from build123d import *

# Parameters (mm, degrees)
F0_W = 64.1248
F0_H = 25.463037
F2_T = -1.27
F4_D = 7.62


with BuildPart() as f1:
    # F0 (on Front) → F1 (revolve)
    with BuildSketch(Plane.XZ):
        with Locations((32.0624, 12.731518)):
            Rectangle(F0_W, F0_H)
    revolve(axis=Axis((0, 0, 5.022522), (0, 0, -1)))

    # F2
    f2_openings = [f1.faces().sort_by_distance(p)[0] for p in [
        (0, 0, 25.463037),
    ]]
    offset(amount=F2_T, openings=f2_openings)

    # F4 (through all)
    with Locations(Plane(origin=(0, 0, 0), x_dir=(1, 0, 0), z_dir=(0, 0, -1))):
        with Locations((0, 0)):
            Hole(F4_D / 2)


solid = f1.part
Geometry: final body of the model. Coordinates: model frame, mm. A direction names the side the tool comes from. Give positions to 0.01 mm unless a question says otherwise; leave off trailing zeros. Order: outer loops, then holes, each group sorted by start corner. A loop starts at its lowest first (then second) coordinate and runs counter-clockwise, first axis right, second up. Notation, with made-up numbers: (-29.5, 10.5) -> (-24.5, 10.5) arc R30 ccw to (-24.5, 47.5) -> close; hole circle Ø1 at (33.5, 68). An arc over 180 degrees is marked (long way). Answer as a JSON object with one key per item and string values.
Q1. Section D-D (y = -17.5). Output: boundary loops of the cut face in (x, z), plus the area to 3 significant figures.
Entries:
{"outline": "(-61.69, 0) -> (61.69, 0) -> (61.69, 25.46) -> (60.37, 25.46) -> (60.37, 1.27) -> (-60.37, 1.27) -> (-60.37, 25.46) -> (-61.69, 25.46) -> close", "area": "221 mm^2"}
Q2. Section A-A (x = 0). Output: boundary loops of the cut face in (y, z), plus the area to 3 significant figures.
Entries:
{"outline": "(-64.12, 0) -> (-3.81, 0) -> (-3.81, 1.27) -> (-62.85, 1.27) -> (-62.85, 25.46) -> (-64.12, 25.46) -> close; (3.81, 0) -> (64.12, 0) -> (64.12, 25.46) -> (62.85, 25.46) -> (62.85, 1.27) -> (3.81, 1.27) -> close", "area": "215 mm^2"}
Q3. Section C-C (z = 13.75). Output: boundary loops of the cut face in (x, y), plus the area to 3 significant figures.
Entries:
{"outline": "circle Ø128.25 at (0, 0); hole circle Ø125.71 at (0, 0)", "area": "507 mm^2"}
Q4. Access query for faces 4 (the flat face through (-13, -1, 1.27)), 5 (the flat face through (1, 13, 0)). Directions: +Z, -Z, +X, -X, +Y, -Y. A direction counts if a zero-diameter tool reaches every point of the face in a straight line with its end or side. Return the directions, or none.
Entries:
{"face 4": "+Z", "face 5": "-Z, +X, -X, +Y, -Y"}
Q5. Draft query along Y for faces 1 (the cylindrical face through (0.83, 3.72, 0.64)), 2 (the flat face through (-42, 47, 25.463)), 3 (the cylindrical face through (-8.35, -63.58, 12.91)). Return one class per face: released by +Y, released by -Y, zero draft, split by the parting line, or undercut.
Entries:
{"face 1": "undercut", "face 2": "zero draft", "face 3": "split by the parting line"}
Q6. First-contact query: pin 1 (12 mm diameter, centred on x = 0, y = 0, fed in from +Z); pin 2 (4 mm diameter, centred on y = 4, z = 21.5, fed in from -X); pin 3 (10 mm diameter, centred on x = -31, z = 6.5, fed in from -Y). Flat tips, straight axial feed; report the tip coordinate or a pass-through.
Entries:
{"pin 1": "stops at z = 1.27", "pin 2": "stops at x = -64.09", "pin 3": "stops at y = -58.62"}
Q7. Material intervals for probe 1 along Y at (x, z) = (0, 7.25); probe 2 along Y at (x, z) = (0, 0.85), sorted ascending.
Entries:
{"probe 1": "y = -64.12 to -62.85, 62.85 to 64.12", "probe 2": "y = -64.12 to -3.81, 3.81 to 64.12"}
